Read the model definition and answer for the solid it produces. Units are mm, in the model's axes. Face numbers are marked on the shaded views. Coordinates: 2 decimals unless noted, no trailing zeros. Write each loop counter-clockwise with the first axis right and the second up, starting at its lowest first coordinate (ties: lowest second). Pieces come first, ordered by that corner, then holes.
Item 1: Determine the mould class of the marked faces 1 and 2 for opening direction Y: released by +Y, released by -Y, zero draft, split by the parting line, or undercut.
Item 2: Each of these flat-tipped pins is pushed along its axis until it touches: P1, Ø4, axis at x = 3.5, z = 52.5, coming from the +Y side; P2, Ø1.5, axis at x = 5, z = 10, coming from the +Y side; P3, Ø6, axis at y = 5.5, z = 49, coming from the -X side. Where does it stop, or does it pass through?
Item 3: Section A-A (z = 36) is taken. Give the vertices of the cut face in (x, y), then the cut area to 3 significant figures.
Item 4: Straight lines are drawn through the part: probe 1 along Y at (x, z) = (0, 64.5); probe 2 along Y at (x, z) = (0, 64.15); probe 3 along Z at (x, y) = (-2, -5.25). For each, find the intervals that lie inside material, in ascending order.
Autodesk Inventor part; units mm, degrees
ref_plane "YZ Plane" through (0, 0, 0) normal (1, 0, 0) x (0, 1, 0)
ref_plane "XZ Plane" through (0, 0, 0) normal (0, 1, 0) x (-1, 0, 0)
ref_plane "XY Plane" through (0, 0, 0) normal (0, 0, 1) x (1, 0, 0)
sketch "Skizze1" plane through (0, 0, 0) normal (0, 1, 0) x (-1, 0, 0)
  line L0 (0, 0) -> (7, 0)
  line L1 (7, 0) -> (7, -0.1)
  line L2 (7, -0.1) -> (8.5, -0.1)
  arc A0 (8.5, -0.1) -> (9, 0.4) centre (8.5, 0.4) ccw
  line L3 (9, 0.4) -> (9, 60.034)
  arc A1 (9, 61.766) -> (9, 60.034) centre (9.5, 60.9) ccw
  line L4 (9, 61.766) -> (9, 64.4)
  arc A2 (9, 64.4) -> (8.5, 64.9) centre (8.5, 64.4) ccw
  line L5 (8.5, 64.9) -> (5, 64.9)
  line L6 (5, 64.9) -> (5, 63.8)
  line L7 (5, 63.8) -> (3, 63.8)
  line L8 (3, 63.8) -> (2.4226, 64.8)
  line L9 (2.4226, 64.8) -> (0, 64.8)
  line L10 (0, 64.8) -> (0, 0)
  dimension "d4" = 18
  dimension "d5" = 1
  dimension "d6" = 19
  dimension "d7" = 0.5
  dimension "d8" = 0.1
  dimension "d9" = 14
  dimension "d10" = 1
  dimension "d11" = 10
  dimension "d12" = 6
  dimension "d13" = 4
  dimension "d14" = 60
  dimension "d17" = 0.1
  dimension "d18" = 65
revolve "Umdrehung1" add sketch "Skizze1" angle 360 about axis through (0, 0, 64.8) along (0, 0, -1)
fillet "Rundung1" radius 2 2 edges at (9, 0, 60.034) (9, 0, 61.766)
equation "\"d17\" = d8"
properties part number "18650"
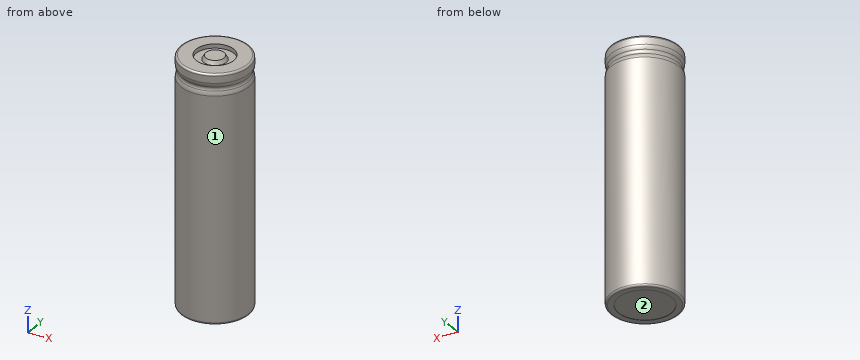
Established:
1. face 1: split by the parting line
1. face 2: undercut
2. P1: stops at y = 8.87
2. P2: stops at y = 7.93
2. P3: stops at x = -8.65
3. outline: circle Ø18 at (0, 0)
3. area: 254 mm2
4. probe 1: y = -8.99 to -5, -2.6 to 2.6, 5 to 8.99
4. probe 2: y = -9 to -5, -2.8 to 2.8, 5 to 9
4. probe 3: z = 0 to 64.9
